from build123d import *

# Parameters (mm, degrees)
F0_W      = 101.6
F0_H      = 609.6
F0_W_2    = 76.2
F0_H_2    = 558.8
F1_DEPTH  = 127
F2_W      = 76.2
F2_H      = 558.8
F3_DEPTH  = 19.05
F4_W      = 76.2
F4_H      = 25.4
F5_DEPTH  = 6.35
F6_W      = 101.6
F6_H      = 101.6
F7_DEPTH  = 25.4
F8_W      = 101.6
F8_H      = 101.6
F9_DEPTH  = 25.4
F3_FACE_W = 76.2
F3_FACE_H = 558.8
F10_DEPTH = 6.35
F11_R     = 6.35
F12_DEPTH = 6.35
F13_R     = 6.35
F14_DEPTH = 12.7
F15_DEPTH = 127


with BuildPart() as f1:
    # F0 (on Top) → F1 (new body)
    with BuildSketch(Plane.XY):
        with Locations((-88.146448, 27.351462)):
            Rectangle(F0_W, F0_H)
        with Locations((-88.146448, 27.351462)):
            Rectangle(F0_W_2, F0_H_2, mode=Mode.SUBTRACT)
    extrude(amount=F1_DEPTH)

    # F2 (on face) → F3 (join)
    with BuildSketch(Plane(origin=(0, 0, 0), x_dir=(1, 0, 0), z_dir=(0, 0, -1))):
        with Locations((-88.146448, -27.351462)):
            Rectangle(F2_W, F2_H)
    extrude(amount=-F3_DEPTH)

    # F4 (on face) → F5 (join)
    with BuildSketch(Plane.XY.offset(127)):
        with Locations((-88.146448, 65.451462)):
            Rectangle(F4_W, F4_H)
        with Locations((-88.146448, -86.948538)):
            Rectangle(F4_W, F4_H)
    extrude(amount=-F5_DEPTH)

    # F6 (on face) → F7 (cut)
    with BuildSketch(Plane.XZ.offset(277.448538)):
        with Locations((-88.146448, 63.5)):
            Rectangle(F6_W, F6_H)
    extrude(amount=-F7_DEPTH, mode=Mode.SUBTRACT)

    # F8 (on face) → F9 (cut)
    with BuildSketch(Plane(origin=(0, 332.151462, 0), x_dir=(-1, 0, 0), z_dir=(0, 1, 0))):
        with Locations((88.146448, 63.5)):
            Rectangle(F8_W, F8_H)
    extrude(amount=-F9_DEPTH, mode=Mode.SUBTRACT)

    # F3_face (on face) → F10 (cut)
    with BuildSketch(Plane(origin=(-88.146448, 27.351462, 19.05), x_dir=(1, 0, 0), z_dir=(0, 0, 1))):
        Rectangle(F3_FACE_W, F3_FACE_H)
    extrude(amount=-F10_DEPTH, mode=Mode.SUBTRACT)

    # F11 (on face) → F12 (cut)
    with BuildSketch(Plane.XY.offset(127)):
        with Locations((-113.546448, 65.451462)):
            Circle(F11_R)
        with Locations((-113.546448, -86.948538)):
            Circle(F11_R)
    extrude(amount=-F12_DEPTH, mode=Mode.SUBTRACT)

    # F13 (on face) → F14 (cut)
    with BuildSketch(Plane.XY.offset(127)):
        with Locations((-119.896448, -264.748538)):
            Circle(F13_R)
        with Locations((-56.396448, -264.748538)):
            Circle(F13_R)
        with Locations((-119.896448, 319.451462)):
            Circle(F13_R)
        with Locations((-56.396448, 319.451462)):
            Circle(F13_R)
    extrude(amount=-F14_DEPTH, mode=Mode.SUBTRACT)

    # F13 (on face) → F15 (cut)
    with BuildSketch(Plane.XY.offset(127)):
        with Locations((-119.896448, 319.451462)):
            Circle(F13_R)
        with Locations((-56.396448, 319.451462)):
            Circle(F13_R)
        with Locations((-119.896448, -264.748538)):
            Circle(F13_R)
        with Locations((-56.396448, -264.748538)):
            Circle(F13_R)
    extrude(amount=-F15_DEPTH, mode=Mode.SUBTRACT)


solid = f1.part
Geometry check sheet. Reference: the model listing, model coordinates, mm. A direction names the side the tool comes from. Give positions to 0.01 mm unless a question says otherwise; leave off trailing zeros. Order: outer loops, then holes, each group sorted by start corner. A loop starts at its lowest first (then second) coordinate and runs counter-clockwise, first axis right, second up.
1. Sectioned sample at B-B (z = 75.5). Record the boundary of the cut face in (x, y), then the cut area to 3 significant figures.
Completed:
outline: (-138.95, -252.05) - (-126.25, -252.05) - (-126.25, 306.75) - (-138.95, 306.75) - close; (-50.05, -252.05) - (-37.35, -252.05) - (-37.35, 306.75) - (-50.05, 306.75) - close
area: 14,200 mm2
2. Scan lines: line 1 (Y direction, x = -87, z = 118); line 2 (X direction, y = 64, z = 41); line 3 (Z direction, x = -108.5, y = -200). Record each from-to range of solid material in increasing order.
Completed:
line 1: y = -277.45 to -252.05, 306.75 to 332.15
line 2: x = -138.95 to -126.25, -50.05 to -37.35
line 3: z = 0 to 12.7
3. Draft check along Z on faces 1 (the face through (-89, 23, 0)), 2 (the face through (-37.346, 23, 63)), 3 (the face through (-89, 66, 120.65)). Enter one of: pulls with the +Z half, pulls with the -Z half, needs draft (parallel to the pull), parting line crosses it, or undercut.
Completed:
face 1: pulls with the -Z half
face 2: needs draft
face 3: undercut
4. Sectioned sample at D-D (x = -55.5). State how many separate pieces and enclosed holes the cut face has, then the cut area to 3 significant figures.
Completed:
separate pieces: 9
enclosed holes: 0
area: 8,070 mm2
5. Access from +Z, -Z, +X, -X, +Y, -Y to the whole of each face (thin tool, end or side, straight path). Record for faces 4 (the face through (-44, -252.049, 64)), 5 (the face through (-89, -87, 120.65)), 6 (the face through (-133, 306.751, 64)), 7 (the face through (-107.68, 63.02, 123.87)).
Completed:
face 4: +X, -X, -Y
face 5: none
face 6: +X, -X, +Y
face 7: +Z
6. Sectioned sample at C-C (y = 26). Record the boundary of the cut face in (x, z), then the cut area to 3 significant figures.
Completed:
outline: (-138.95, 0) - (-37.35, 0) - (-37.35, 127) - (-50.05, 127) - (-50.05, 12.7) - (-126.25, 12.7) - (-126.25, 127) - (-138.95, 127) - close
area: 4,190 mm2
7. Depth check by flat-ended pin: pin 1 (10 mm diameter, centred on x = -55, z = 61, fed in from -Y); pin 2 (6 mm diameter, centred on x = -86.5, y = -165.5, fed in from +Z); pin 3 (3 mm diameter, centred on x = -50, z = 76.5, fed in from +Y). Enter the tip coordinate at first touch or a pass-through.
Completed:
pin 1: stops at y = -252.05
pin 2: stops at z = 12.7
pin 3: stops at y = 306.75
8. Sectioned sample at A-A (x = -88.5). Record the boundary of the cut face in (y, z), then the cut area to 3 significant figures.
Completed:
outline: (-277.45, 0) - (332.15, 0) - (332.15, 12.7) - (-277.45, 12.7) - close; (-277.45, 114.3) - (-252.05, 114.3) - (-252.05, 127) - (-277.45, 127) - close; (-99.65, 120.65) - (-74.25, 120.65) - (-74.25, 127) - (-99.65, 127) - close; (52.75, 120.65) - (78.15, 120.65) - (78.15, 127) - (52.75, 127) - close; (306.75, 114.3) - (332.15, 114.3) - (332.15, 127) - (306.75, 127) - close
area: 8,710 mm2
